from build123d import *

# Parameters (mm, degrees)
F0_R      = 10
F0_R_2    = 8.5
F1_DEPTH  = 50
F2_R      = 8.5
F3_DEPTH  = 1.5
F4_R      = 2.5
F5_DEPTH  = 12.5
F7_R      = 10
F7_R_2    = 9.75
F8_DEPTH  = 0.5
F10_R     = 10
F10_R_2   = 9.5
F11_DEPTH = 0.5


# Not quite as in the source:
# - a pattern or mirror of a feature is missing from the dataset's text; its kind, count and spacing are read off the source's solid


with BuildPart() as f1:
    # F0 (on Top) → F1 (new body, symmetric)
    with BuildSketch(Plane.XY):
        Circle(F0_R)
        Circle(F0_R_2, mode=Mode.SUBTRACT)
    extrude(amount=F1_DEPTH, both=True)

    # F2 (on face) → F3 (join)
    with BuildSketch(Plane.XY.offset(50)):
        Circle(F2_R)
    f3 = extrude(amount=-F3_DEPTH)

    # F3_copies: F3 across plane
    add(f3.mirror(Plane(origin=(0, 0, 0), x_dir=(-1, 0, 0), z_dir=(0, 0, -1))))

    # F4 (on Right) → F5 (cut, symmetric)
    with BuildSketch(Plane.YZ):
        with Locations((0, -20)):
            Circle(F4_R)
    extrude(amount=F5_DEPTH, both=True, mode=Mode.SUBTRACT)

    # F7 (on offset) → F8 (cut, symmetric)
    with BuildSketch(Plane.XY.offset(45)):
        Circle(F7_R)
        Circle(F7_R_2, mode=Mode.SUBTRACT)
    extrude(amount=F8_DEPTH, both=True, mode=Mode.SUBTRACT)

    # F10 (on face) → F11 (cut, symmetric)
    with BuildSketch(Plane(origin=(0, 0, -35), x_dir=(1, 0, 0), z_dir=(0, 0, -1))):
        Circle(F10_R)
        Circle(F10_R_2, mode=Mode.SUBTRACT)
    extrude(amount=F11_DEPTH, both=True, mode=Mode.SUBTRACT)


solid = f1.part
Geometry check sheet. Reference: the model listing, model coordinates, mm. A direction names the side the tool comes from. Coordinates: 2 decimals unless noted, no trailing zeros. Order: outer loops, then holes, each group sorted by start corner. A loop starts at its lowest first (then second) coordinate and runs counter-clockwise, first axis right, second up. Notation, with made-up numbers: (-30, 77.25) - (25, 77.25) arc R11 cw to (25, 96.25) - close; hole circle Ø5 at (-31, 25). An arc over 180 degrees is marked (long way). Answer in a Markdown table with one row per item. Add a question column.
1) Cross-section at D-D, the plane z = 17. Record the cut outline in (x, y).
2) Release check for a two-part mould opening along Z. For faces 3 (the cylindrical face through (9.54, 3, 5.55)), 4 (the flat face through (0, 0, 50)), 5 (the flat face through (0, 0, -50)), 6 (the cylindrical face through (-1.269, 9.667, 44.993)) record: +Z half, -Z half, draft (parallel to the pull), parting line (faces both ways), or undercut.
3) Cross-section at C-C, the plane x = 0. Record the cut outline in (y, z), then the cut area to 4 significant figures.
4) Gauge pin test, flat ends, axial feed: P1, Ø3, axis at y = 1.5, z = -4, coming from the +X side; P2, Ø4, axis at y = -6, z = -17, coming from the +X side; P3, Ø5, axis at y = -4, z = 31, coming from the -X side; P4, Ø4.5, axis at y = 0, z = -20, coming from the -X side. Record the tip position at first contact, or that the pin passes through.
5) Set-up check for faces 1 (the cylindrical face through (-9.05, 2.31, -20.96)), 2 (the cylindrical face through (4.38, 8.43, -34.99)): record each of +Z, -Z, +X, -X, +Y, -Y from which the full face is reachable in a straight line by a thin tool's end or side.
6) Material ranges on line 1 along Z through (x, y) = (9.55, 0); line 2 along Z through (x, y) = (4.5, -6.75); line 3 along Z through (x, y) = (9, -3.5), recorded low to high. Write a range as [from, to].
7) Cross-section at B-B, the plane z = -20. Record the cut outline in (x, y).
Check result:
| question | item | result |
|---|---|---|
| 1 | outline | circle Ø20 at (0, 0); hole circle Ø17 at (0, 0) |
| 2 | face 3 | draft |
| 2 | face 4 | +Z half |
| 2 | face 5 | -Z half |
| 2 | face 6 | undercut |
| 3 | outline | (-10, -50) - (10, -50) - (10, -35.5) - (9.5, -35.5) - (9.5, -34.5) - (10, -34.5) - (10, 44.5) - (9.75, 44.5) - (9.75, 45.5) - (10, 45.5) - (10, 50) - (-10, 50) - (-10, 45.5) - (-9.75, 45.5) - (-9.75, 44.5) - (-10, 44.5) - (-10, -34.5) - (-9.5, -34.5) - (-9.5, -35.5) - (-10, -35.5) - close; hole (-8.5, -48.5) - (8.5, -48.5) - (8.5, 48.5) - (-8.5, 48.5) - close |
| 3 | area | 349.5 mm² |
| 4 | P1 | stops at x = 10 |
| 4 | P2 | stops at x = 9.17 |
| 4 | P3 | stops at x = -9.89 |
| 4 | P4 | passes through |
| 5 | face 1 | +X, -X |
| 5 | face 2 | none |
| 6 | line 1 | z = [-50, -35.5], [-34.5, -22.5], [-17.5, 50] |
| 6 | line 2 | z = [-50, -48.5], [48.5, 50] |
| 6 | line 3 | z = [-50, -35.5], [-34.5, 50] |
| 7 | outline | (-9.68, -2.5) arc R10 ccw to (9.68, -2.5) - (8.12, -2.5) arc R8.5 cw to (-8.12, -2.5) - close; (-9.68, 2.5) - (-8.12, 2.5) arc R8.5 cw to (8.12, 2.5) - (9.68, 2.5) arc R10 ccw to start |
